from build123d import *

# Parameters (mm, degrees)
SKETCH_1_R          = 9
EXTRUDE_1_DEPTH     = 1
SKETCH_2_R          = 6
EXTRUDE_2_DEPTH     = 6.5
SKETCH_3_R          = 9
EXTRUDE_3_DEPTH     = 1
SKETCH_4_R          = 1.5
CUT_EXTRUDE_1_DEPTH = 9.5
CUT_EXTRUDE_2_DEPTH = 6.5


with BuildPart() as part:
    # 草图1 → 凸台-拉伸1 (new body)
    with BuildSketch(Plane(origin=(0, 0, 0), x_dir=(1, 0, 0), z_dir=(0, 1, 0))):
        Circle(SKETCH_1_R)
    extrude(amount=EXTRUDE_1_DEPTH)

    # 草图2 → 凸台-拉伸2 (add)
    with BuildSketch(Plane(origin=(0, 1, 0), x_dir=(1, 0, 0), z_dir=(0, 1, 0))):
        Circle(SKETCH_2_R)
    extrude(amount=EXTRUDE_2_DEPTH)

    # 草图3 → 凸台-拉伸3 (add)
    with BuildSketch(Plane(origin=(0, 7.5, 0), x_dir=(1, 0, 0), z_dir=(0, 1, 0))):
        Circle(SKETCH_3_R)
    extrude(amount=EXTRUDE_3_DEPTH)

    # 草图4 → 切除-拉伸1 (cut, through all)
    with BuildSketch(Plane(origin=(0, 8.5, 0), x_dir=(1, 0, 0), z_dir=(0, 1, 0))):
        Circle(SKETCH_4_R)
    extrude(amount=-CUT_EXTRUDE_1_DEPTH, mode=Mode.SUBTRACT)

    # 草图5 → 切除-拉伸2 (cut)
    with BuildSketch(Plane(origin=(0, 1, 0), x_dir=(1, 0, 0), z_dir=(0, 1, 0))):
        with BuildLine():
            Line((-6, 0), (-4.984088538, 0.398574263))
            ThreePointArc((-4.984088538, 0.398574263), (-4.96506054, 0.590062568), (-4.938678327, 0.780676876))
            Line((-4.938678327, 0.780676876), (-5.83314158, 1.40515455))
            ThreePointArc((-5.83314158, 1.40515455), (-5.958139369, 0.707513435), (-6, 0))
        make_face()
        with BuildLine():
            Line((-5.981863946, -0.466158487), (-4.938204626, -0.783667703))
            ThreePointArc((-4.938204626, -0.783667703), (-4.904392542, -0.973105234), (-4.863316103, -1.161101409))
            Line((-4.863316103, -1.161101409), (-5.706339098, -1.854101966))
            ThreePointArc((-5.706339098, -1.854101966), (-5.885160947, -1.168281057), (-5.981863946, -0.466158487))
        make_face()
        with BuildLine():
            Line((-5.706339098, 1.854101966), (-4.616983661, 1.91923471))
            ThreePointArc((-4.616983661, 1.91923471), (-4.539713819, 2.095470935), (-4.455719783, 2.268603363))
            Line((-4.455719783, 2.268603363), (-5.113430674, 3.13892127))
            ThreePointArc((-5.113430674, 3.13892127), (-5.447893597, 2.514051583), (-5.706339098, 1.854101966))
        make_face()
        with BuildLine():
            Line((-4.854101966, 3.526711514), (-3.797936255, 3.252027091))
            ThreePointArc((-3.797936255, 3.252027091), (-3.669988279, 3.395760008), (-3.536604341, 3.534463146))
            Line((-3.536604341, 3.534463146), (-3.893181547, 4.565428506))
            ThreePointArc((-3.893181547, 4.565428506), (-4.404370041, 4.074496845), (-4.854101966, 3.526711514))
        make_face()
        with BuildLine():
            Line((-3.526711514, 4.854101966), (-2.607120386, 4.266488403))
            ThreePointArc((-2.607120386, 4.266488403), (-2.441018717, 4.36364843), (-2.271301426, 4.454345051))
            Line((-2.271301426, 4.454345051), (-2.291840684, 5.545039791))
            ThreePointArc((-2.291840684, 5.545039791), (-2.929716059, 5.236101967), (-3.526711514, 4.854101966))
        make_face()
        with BuildLine():
            Line((-1.854101966, 5.706339098), (-1.161101409, 4.863316103))
            ThreePointArc((-1.161101409, 4.863316103), (-0.973105234, 4.904392542), (-0.783667703, 4.938204626))
            Line((-0.783667703, 4.938204626), (-0.466158487, 5.981863946))
            ThreePointArc((-0.466158487, 5.981863946), (-1.168281057, 5.885160947), (-1.854101966, 5.706339098))
        make_face()
        with BuildLine():
            Line((0, 6), (0.398574263, 4.984088538))
            ThreePointArc((0.398574263, 4.984088538), (0.590062568, 4.96506054), (0.780676876, 4.938678327))
            Line((0.780676876, 4.938678327), (1.40515455, 5.83314158))
            ThreePointArc((1.40515455, 5.83314158), (0.707513435, 5.958139369), (0, 6))
        make_face()
        with BuildLine():
            Line((1.854101966, 5.706339098), (1.91923471, 4.616983661))
            ThreePointArc((1.91923471, 4.616983661), (2.095470935, 4.539713819), (2.268603363, 4.455719783))
            Line((2.268603363, 4.455719783), (3.13892127, 5.113430674))
            ThreePointArc((3.13892127, 5.113430674), (2.514051583, 5.447893597), (1.854101966, 5.706339098))
        make_face()
        with BuildLine():
            Line((3.526711514, 4.854101966), (3.252027091, 3.797936255))
            ThreePointArc((3.252027091, 3.797936255), (3.395760008, 3.669988279), (3.534463146, 3.536604341))
            Line((3.534463146, 3.536604341), (4.565428506, 3.893181547))
            ThreePointArc((4.565428506, 3.893181547), (4.074496845, 4.404370041), (3.526711514, 4.854101966))
        make_face()
        with BuildLine():
            Line((4.854101966, 3.526711514), (4.266488403, 2.607120386))
            ThreePointArc((4.266488403, 2.607120386), (4.36364843, 2.441018717), (4.454345051, 2.271301426))
            Line((4.454345051, 2.271301426), (5.545039791, 2.291840684))
            ThreePointArc((5.545039791, 2.291840684), (5.236101967, 2.929716059), (4.854101966, 3.526711514))
        make_face()
        with BuildLine():
            Line((5.706339098, 1.854101966), (4.863316103, 1.161101409))
            ThreePointArc((4.863316103, 1.161101409), (4.904392542, 0.973105234), (4.938204626, 0.783667703))
            Line((4.938204626, 0.783667703), (5.981863946, 0.466158487))
            ThreePointArc((5.981863946, 0.466158487), (5.885160947, 1.168281057), (5.706339098, 1.854101966))
        make_face()
        with BuildLine():
            Line((6, 0), (4.984088538, -0.398574263))
            ThreePointArc((4.984088538, -0.398574263), (4.96506054, -0.590062568), (4.938678327, -0.780676876))
            Line((4.938678327, -0.780676876), (5.83314158, -1.40515455))
            ThreePointArc((5.83314158, -1.40515455), (5.958139369, -0.707513435), (6, 0))
        make_face()
        with BuildLine():
            Line((5.706339098, -1.854101966), (4.616983661, -1.91923471))
            ThreePointArc((4.616983661, -1.91923471), (4.539713819, -2.095470935), (4.455719783, -2.268603363))
            Line((4.455719783, -2.268603363), (5.113430674, -3.13892127))
            ThreePointArc((5.113430674, -3.13892127), (5.447893597, -2.514051583), (5.706339098, -1.854101966))
        make_face()
        with BuildLine():
            Line((4.854101966, -3.526711514), (3.797936255, -3.252027091))
            ThreePointArc((3.797936255, -3.252027091), (3.669988279, -3.395760008), (3.536604341, -3.534463146))
            Line((3.536604341, -3.534463146), (3.893181547, -4.565428506))
            ThreePointArc((3.893181547, -4.565428506), (4.404370041, -4.074496845), (4.854101966, -3.526711514))
        make_face()
        with BuildLine():
            Line((3.526711514, -4.854101966), (2.607120386, -4.266488403))
            ThreePointArc((2.607120386, -4.266488403), (2.441018717, -4.36364843), (2.271301426, -4.454345051))
            Line((2.271301426, -4.454345051), (2.291840684, -5.545039791))
            ThreePointArc((2.291840684, -5.545039791), (2.929716059, -5.236101967), (3.526711514, -4.854101966))
        make_face()
        with BuildLine():
            Line((1.854101966, -5.706339098), (1.161101409, -4.863316103))
            ThreePointArc((1.161101409, -4.863316103), (0.973105234, -4.904392542), (0.783667703, -4.938204626))
            Line((0.783667703, -4.938204626), (0.466158487, -5.981863946))
            ThreePointArc((0.466158487, -5.981863946), (1.168281057, -5.885160947), (1.854101966, -5.706339098))
        make_face()
        with BuildLine():
            Line((0, -6), (-0.398574263, -4.984088538))
            ThreePointArc((-0.398574263, -4.984088538), (-0.590062568, -4.96506054), (-0.780676876, -4.938678327))
            Line((-0.780676876, -4.938678327), (-1.40515455, -5.83314158))
            ThreePointArc((-1.40515455, -5.83314158), (-0.707513435, -5.958139369), (0, -6))
        make_face()
        with BuildLine():
            Line((-1.854101966, -5.706339098), (-1.91923471, -4.616983661))
            ThreePointArc((-1.91923471, -4.616983661), (-2.095470935, -4.539713819), (-2.268603363, -4.455719783))
            Line((-2.268603363, -4.455719783), (-3.13892127, -5.113430674))
            ThreePointArc((-3.13892127, -5.113430674), (-2.514051583, -5.447893597), (-1.854101966, -5.706339098))
        make_face()
        with BuildLine():
            Line((-3.526711514, -4.854101966), (-3.252027091, -3.797936255))
            ThreePointArc((-3.252027091, -3.797936255), (-3.395760008, -3.669988279), (-3.534463146, -3.536604341))
            Line((-3.534463146, -3.536604341), (-4.565428506, -3.893181547))
            ThreePointArc((-4.565428506, -3.893181547), (-4.074496845, -4.404370041), (-3.526711514, -4.854101966))
        make_face()
        with BuildLine():
            Line((-4.854101966, -3.526711514), (-4.266488403, -2.607120386))
            ThreePointArc((-4.266488403, -2.607120386), (-4.36364843, -2.441018717), (-4.454345051, -2.271301426))
            Line((-4.454345051, -2.271301426), (-5.545039791, -2.291840684))
            ThreePointArc((-5.545039791, -2.291840684), (-5.236101967, -2.929716059), (-4.854101966, -3.526711514))
        make_face()
    extrude(amount=CUT_EXTRUDE_2_DEPTH, mode=Mode.SUBTRACT)


solid = part.part
Geometry check sheet. Reference: the model listing, model coordinates, mm. A direction names the side the tool comes from. Round coordinates to 2 decimals unless told otherwise and drop trailing zeros. Order: outer loops, then holes, each group sorted by start corner. A loop starts at its lowest first (then second) coordinate and runs counter-clockwise, first axis right, second up. Notation, with made-up numbers: M -0.5,14.25 L 41.5,14.25 A29 cw 41.5,46.25 Z; hole C 79.5,56.5 d5. An arc over 180 degrees is marked long. Answer in a Markdown table with one row per item. Add a question column.
Item 1: Material ranges on L1, parallel to Y at x = 5, z = 4.25; L2, parallel to Z at x = 5.25, y = 3.5; L3, parallel to X at y = 6.75, z = -1, recorded low to high. Write a range as [from, to].
Item 2: Sectioned sample at B-B, the plane x = 6.75. Enter the section's corners in (y, z).
Item 3: Set-up check for faces 3 (the face through (-0.63, 4.2, -5.45)), 4 (the face through (4, 1, 4)), 5 (the face through (-3.71, 4.2, -4.04)), 6 (the face through (-2.7, 4.2, 4.78)), 7 (the face through (4.56, 4.2, -3.07)): record each of +Z, -Z, +X, -X, +Y, -Y from which the full face is reachable in a straight line by a thin tool's end or side.
Item 4: Draft check along Y on faces 1 (the face through (0.196, 4.204, -5.499)), 2 (the face through (-1.172, 7.993, -8.923)). Enter one of: released by +Y, released by -Y, zero draft, split by the parting line, or undercut.
Item 5: Sectioned sample at A-A, the plane z = 7. Enter the section's corners in (x, y).
Item 6: Depth check by flat-ended pin: pin 1 Ø4 at (x, y) = (0.5, 6) entering from +Z; pin 2 Ø4 at (x, y) = (3, 1.5) entering from -Z; pin 3 Ø4 at (x, y) = (6, 3.5) entering from -Z; pin 4 Ø1 at (x, y) = (-6, 5) entering from -Z. Enter the tip coordinate at first touch or a pass-through.
Filled in:
| question | item | result |
|---|---|---|
| 1 | L1 | y = [0, 1], [7.5, 8.5] |
| 1 | L2 | z = [-2.29, -1.48], [-0.69, 0.29], [1, 1.88] |
| 1 | L3 | x = [-5.25, -1.12], [1.12, 4.9] |
| 2 | outline | M 0,-5.95 L 1,-5.95 L 1,5.95 L 0,5.95 Z; M 7.5,-5.95 L 8.5,-5.95 L 8.5,5.95 L 7.5,5.95 Z |
| 3 | face 3 | -Z |
| 3 | face 4 | none |
| 3 | face 5 | -X |
| 3 | face 6 | +Z |
| 3 | face 7 | +X |
| 4 | face 1 | undercut |
| 4 | face 2 | zero draft |
| 5 | outline | M -5.66,0 L 5.66,0 L 5.66,1 L -5.66,1 Z; M -5.66,7.5 L 5.66,7.5 L 5.66,8.5 L -5.66,8.5 Z |
| 6 | pin 1 | stops at z = 9 |
| 6 | pin 2 | stops at z = -8.94 |
| 6 | pin 3 | stops at z = -3.89 |
| 6 | pin 4 | stops at z = -1.87 |
